Design review of the part built by this model. Coordinates are the model's own, in mm. Face numbers are marked on the shaded views. A direction names the side the tool comes from. Give positions to 0.01 mm unless a question says otherwise; leave off trailing zeros. Use a Markdown table: item, result. Add a question column.
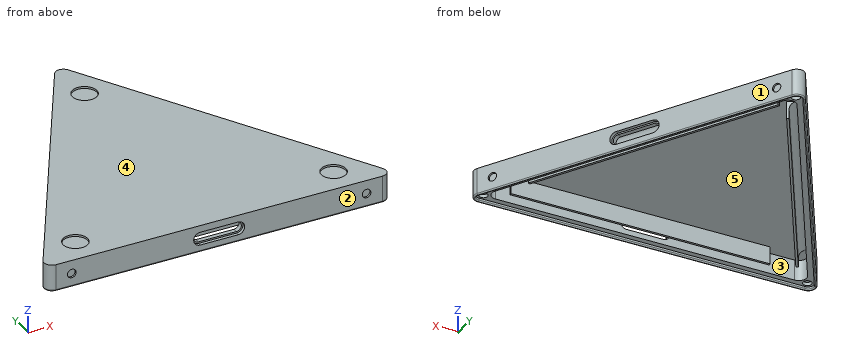
```python
from build123d import *

# Parameters (mm, degrees)
BOSS_EXTRU_1_DEPTH      = 15
BOSS_EXTRU_2_DEPTH      = 2
ESQUISSE3_W             = 164.930853143
ESQUISSE3_H             = 1.4
BOSS_EXTRU_3_DEPTH      = 11
ENL_V_MAT_EXTRU_1_DEPTH = 2.1
ENL_V_MAT_EXTRU_2_REACH = 232.446
CONG_1_R                = 5
ESQUISSE6_R             = 7.75
ENL_V_MAT_EXTRU_3_DEPTH = 1.24
ESQUISSE7_R             = 2.75
ENL_V_MAT_EXTRU_4_DEPTH = 1.24
CONG_2_R                = 5
ENL_V_MAT_EXTRU_6_DEPTH = 2
ESQUISSE8_R             = 2.75
ENL_V_MAT_EXTRU_5_DEPTH = 4.1
CONG_3_R                = 0.75


with BuildPart() as part:
    # Esquisse1 → Boss.-Extru.1 (new body)
    with BuildSketch(Plane.XY):
        Polygon((-169.71822613, -51.377911564), (-57.21822613, 143.477804287), (55.28177387, -51.377911564), align=None)
        Polygon((46.621519833, -46.377911564), (-161.057972092, -46.377911564), (-57.21822613, 133.477804287), align=None, mode=Mode.SUBTRACT)
    extrude(amount=BOSS_EXTRU_1_DEPTH)

    # Esquisse2 → Boss.-Extru.2 (add)
    with BuildSketch(Plane.XY.offset(15)):
        Polygon((-57.21822613, 143.477804287), (-169.71822613, -51.377911564), (55.28177387, -51.377911564), align=None)
    extrude(amount=BOSS_EXTRU_2_DEPTH)

    # Esquisse3 → Boss.-Extru.3 (add)
    with BuildSketch(Plane(origin=(0, 0, 15), x_dir=(-1, 0, 0), z_dir=(0, 0, -1))):
        Polygon((53.949011072, 117.815357706), (-28.5164155, -25.018950984), (-27.303979934, -25.718950984), (55.161446637, 117.115357706), align=None)
        Polygon((149.019751584, -35.527102012), (147.807316018, -36.227102012), (65.341889447, 106.607206677), (66.554325012, 107.307206677), align=None)
        with Locations((51.042590893, -40.677911564)):
            Rectangle(ESQUISSE3_W, ESQUISSE3_H)
    extrude(amount=BOSS_EXTRU_3_DEPTH)

    # Esquisse4 → Enlèv. mat.-Extru.1 (cut)
    with BuildSketch(Plane(origin=(19.214042099, 11.093232378, 0), x_dir=(0, 0, -1), z_dir=(0.8660254037844387, 0.5000000000000001, 0))):
        with BuildLine():
            Line((-12.65, 52.464536457), (-12.65, 28.264536457))
            ThreePointArc((-12.65, 28.264536457), (-8.5, 24.114536457), (-4.35, 28.264536457))
            Line((-4.35, 28.264536457), (-4.35, 52.464536457))
            ThreePointArc((-4.35, 52.464536457), (-8.5, 56.614536457), (-12.65, 52.464536457))
        make_face()
    enl_v_mat_extru_1 = extrude(amount=-ENL_V_MAT_EXTRU_1_DEPTH, mode=Mode.SUBTRACT)

    # Esquisse5 → Enlèv. mat.-Extru.2 (cut, up to next)
    with BuildSketch(Plane(origin=(17.395388751, 10.043232378, 0), x_dir=(0, 0, -1), z_dir=(0.8660254037844386, 0.5000000000000003, 0)), mode=Mode.PRIVATE) as enl_v_mat_extru_2_sk1:
        with BuildLine():
            Line((-11.65, 52.464536457), (-11.65, 28.264536457))
            ThreePointArc((-11.65, 28.264536457), (-8.5, 25.114536457), (-5.35, 28.264536457))
            Line((-5.35, 28.264536457), (-5.35, 52.464536457))
            ThreePointArc((-5.35, 52.464536457), (-8.5, 55.614536457), (-11.65, 52.464536457))
        make_face()
    enl_v_mat_extru_2_tool1 = extrude(enl_v_mat_extru_2_sk1.sketch, amount=-ENL_V_MAT_EXTRU_2_REACH, mode=Mode.PRIVATE) & part.part
    enl_v_mat_extru_2 = enl_v_mat_extru_2_tool1.solids().sort_by_distance((-2.786879, 44.999946, 8.5))[0]
    add(enl_v_mat_extru_2, mode=Mode.SUBTRACT)

    # Congé1
    cong_1_edges = [part.edges().sort_by_distance(p)[0] for p in [
        (46.621519833, -46.377911564, 7.5),
        (-57.21822613, 133.477804287, 7.5),
        (-161.057972092, -46.377911564, 7.5),
        (-169.71822613, -51.377911564, 8.5),
        (-57.21822613, 143.477804287, 8.5),
        (55.28177387, -51.377911564, 8.5),
    ]]
    fillet(cong_1_edges, radius=CONG_1_R)

    # Symétrie1: Enlèv. mat.-Extru.1, Enlèv. mat.-Extru.2 across plane
    add(enl_v_mat_extru_1.mirror(Plane(origin=(-8.426844836, -14.595723404, 0), x_dir=(0, 0, 1), z_dir=(0.5000000000000001, 0.8660254037844386, 0))), mode=Mode.SUBTRACT)
    add(enl_v_mat_extru_2.mirror(Plane(origin=(-8.426844836, -14.595723404, 0), x_dir=(0, 0, 1), z_dir=(0.5000000000000001, 0.8660254037844386, 0))), mode=Mode.SUBTRACT)

    # Esquisse6 → Enlèv. mat.-Extru.3 (cut)
    with BuildSketch(Plane.XY.offset(17)):
        with Locations((-57.21822613, 108.477804287)):
            Circle(ESQUISSE6_R)
        with Locations(Location((-139.407336997, -33.877911564, 0), (0, 0, 180))):
            Circle(ESQUISSE6_R)
        with Locations((24.970884738, -33.877911564)):
            Circle(ESQUISSE6_R)
    extrude(amount=-ENL_V_MAT_EXTRU_3_DEPTH, mode=Mode.SUBTRACT)

    # Esquisse7 → Enlèv. mat.-Extru.4 (cut)
    with BuildSketch(Plane.XZ.offset(51.377911564)):
        with Locations((36.621519833, 8.5)):
            Circle(ESQUISSE7_R)
        with Locations(Location((-151.057972092, 8.5, 0), (0, 0, 180))):
            Circle(ESQUISSE7_R)
    enl_v_mat_extru_4 = extrude(amount=-ENL_V_MAT_EXTRU_4_DEPTH, mode=Mode.SUBTRACT)

    # Symétrie2: Enlèv. mat.-Extru.4 across plane
    add(enl_v_mat_extru_4.mirror(Plane(origin=(-8.426844836, -14.595723404, 0), x_dir=(0, 0, 1), z_dir=(0.5000000000000001, 0.8660254037844386, 0))), mode=Mode.SUBTRACT)

    # Symétrie3: Enlèv. mat.-Extru.4 across plane
    add(enl_v_mat_extru_4.mirror(Plane(origin=(-20.182268228, 34.956713983, 0), x_dir=(0, 0, 1), z_dir=(0.5000000000000001, -0.8660254037844387, 0))), mode=Mode.SUBTRACT)

    # Congé2
    cong_2_edges = [part.edges().sort_by_distance(p)[0] for p in [
        (-12.716297786, 46.398203361, 15),
        (-107.787038298, 35.890052333, 15),
        (-51.042590892, -41.377911564, 15),
    ]]
    fillet(cong_2_edges, radius=CONG_2_R - 0.0001)  # a hair under: the kernel refuses the full size

    # Esquisse9 → Enlèv. mat.-Extru.6 (cut)
    with BuildSketch(Plane(origin=(0, 0, 0), x_dir=(-1, 0, 0), z_dir=(0, 0, -1))):
        with BuildLine():
            Line((164.089061005, -44.627911564), (60.249315043, 135.227804287))
            ThreePointArc((60.249315043, 135.227804287), (57.21822613, 136.977804287), (54.187137216, 135.227804287))
            Line((54.187137216, 135.227804287), (-49.652608746, -44.627911564))
            ThreePointArc((-49.652608746, -44.627911564), (-49.652608746, -48.127911564), (-46.621519833, -49.877911564))
            Line((-46.621519833, -49.877911564), (161.057972092, -49.877911564))
            ThreePointArc((161.057972092, -49.877911564), (164.089061005, -48.127911564), (164.089061005, -44.627911564))
        make_face()
    extrude(amount=-ENL_V_MAT_EXTRU_6_DEPTH, mode=Mode.SUBTRACT)

    # Esquisse8 → Enlèv. mat.-Extru.5 (cut)
    with BuildSketch(Plane(origin=(0, 0, 0), x_dir=(-1, 0, 0), z_dir=(0, 0, -1))):
        with Locations((-45.914902423, -45.969945813)):
            Circle(ESQUISSE8_R)
        with Locations((57.21822613, 132.661872783)):
            Circle(ESQUISSE8_R)
        with Locations((160.351354682, -45.969945813)):
            Circle(ESQUISSE8_R)
    extrude(amount=-ENL_V_MAT_EXTRU_5_DEPTH, mode=Mode.SUBTRACT)

    # Congé3
    cong_3_edges = [part.edges().sort_by_distance(p)[0] for p in [
        (-113.46822613, 46.049946361, 0),
        (-57.21822613, -51.377911564, 0),
        (-0.96822613, 46.049946361, 0),
        (50.951646852, -48.877911564, 0),
        (-165.388099111, -48.877911564, 0),
        (-57.21822613, 138.477804287, 0),
        (-112.169188024, 45.299946361, 0),
        (-2.267264235, 45.299946361, 0),
        (-57.21822613, -49.877911564, 0),
    ]]
    fillet(cong_3_edges, radius=CONG_3_R - 0.0001)  # a hair under: the kernel refuses the full size


solid = part.part
```
(1) Wall thickness on L1, parallel to Y at x = -17, z = 4.25; L2, parallel to Y at x = -67, z = 4.75; L3, parallel to X at y = -23, z = 9: over which ranges is each line inside the solid? List them lowest first.
(2) Machinability: for the marked faces 4 and 5, which of the approach directions +Z, -Z, +X, -X, +Y, -Y give a long, thin tool a straight path to every point of the face, cutting with its end or side? Answer none if there is none.
(3) The part is to be moulded in two halves that separate along X. For the marked faces 1, 2 and 3, say which applies: released by +X, released by -X, zero draft, split by the parting line, or undercut.
(4) For pin 1 (1.5 mm diameter, centred on x = -46, z = 8, fed in from -Y); pin 2 (14 mm diameter, centred on x = -139.41, y = -33.88, fed in from -Z); pin 3 (4.5 mm diameter, centred on x = -160.5, y = -47, fed in from -Z); pin 4 (4 mm diameter, centred on x = -91.5, y = 85, fed in from +Z), all flat-tipped, find the tip position at first contact; note any pin that passes through.
From the geometry:
| question | item | result |
|---|---|---|
| 1 | L1 | y = -51.38 to -46.38, -41.38 to -39.98, 51.02 to 53.82, 63.82 to 73.82 |
| 1 | L2 | y = -49.28 to -46.38, -41.38 to -39.98, 103.74 to 106.54, 116.54 to 126.54 |
| 1 | L3 | x = -153.33 to -147.56, -141.79 to -140.17, 25.73 to 27.35, 33.12 to 38.9 |
| 2 | face 4 | +Z, +X, -X, +Y, -Y |
| 2 | face 5 | -Z |
| 3 | face 1 | released by +X |
| 3 | face 2 | zero draft |
| 3 | face 3 | undercut |
| 4 | pin 1 | stops at y = -41.38 |
| 4 | pin 2 | stops at z = 4 |
| 4 | pin 3 | stops at z = 2 |
| 4 | pin 4 | stops at z = 17 |
